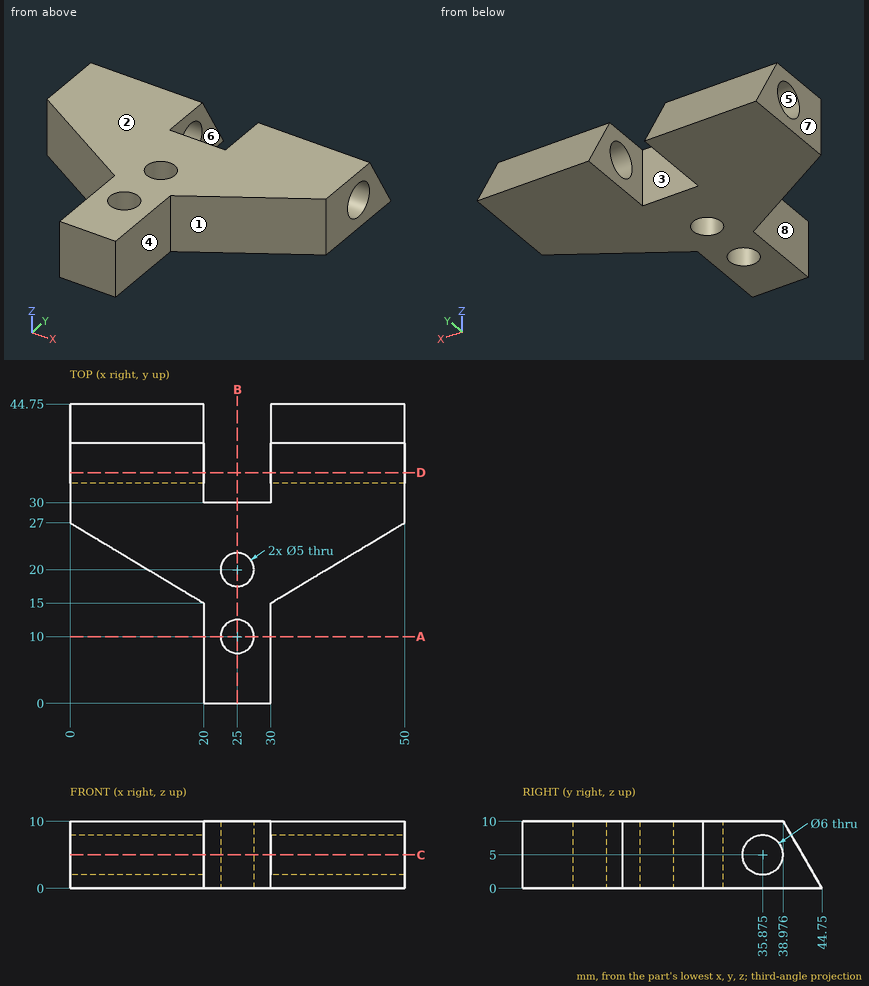
Study the drawing (mm; zero at the part's minimum x, y, z) and answer. A direction names the side the tool comes from. Round coordinates to 2 decimals unless told otherwise and drop trailing zeros. Write each loop counter-clockwise with the first axis right and the second up, starting at its lowest first coordinate (ties: lowest second). Pieces come first, ordered by that corner, then holes.
Q1. A tool of negligible diameter and unlimited length cuts with its end or side. For the marked faces 4, 5, 6, 7 and 8, from which of +Z, -Z, +X, -X, +Y, -Y can it reach the whole face along a straight path? Write none if from no direction.
Values:
face 4: +Z, -Z, +X, -Y
face 5: +X, -X
face 6: +Z, -Z, +Y
face 7: +Z, -Z, -X, +Y, -Y
face 8: +Z, -Z, -X, -Y
Q2. The mould has two halves that part along X. Classify the marked faces 1, 2 and 3: released by +X, released by -X, zero draft, split by the parting line, or undercut.
Values:
face 1: released by +X
face 2: zero draft
face 3: undercut
Q3. Find section C-C on z = 5. Determine the outline of the cut face in (x, y) (1 decimal).
Values:
outline: (0, 27) - (20, 15) - (20, 0) - (30, 0) - (30, 15) - (50, 27) - (50, 32.9) - (30, 32.9) - (30, 30) - (20, 30) - (20, 32.9) - (0, 32.9) - close; (0, 38.9) - (20, 38.9) - (20, 41.9) - (0, 41.9) - close; (30, 38.9) - (50, 38.9) - (50, 41.9) - (30, 41.9) - close; hole circle Ø5 at (25, 10); hole circle Ø5 at (25, 20)
Q4. Flat-ended cylindrical pins translate along their axes: P1, Ø3, axis at x = 23.5, z = 5, coming from the +Y side; P2, Ø2, axis at y = 15, z = 8.5, coming from the +X side (1 decimal); P3, Ø5, axis at y = 10.5, z = 2.5, coming from the +X side. Find the tip coordinate at first contact, or state that the pin passes through.
Values:
P1: stops at y = 30
P2: stops at x = 31.7
P3: stops at x = 30
Q5. Find section D-D on y = 34.5. Determine the outline of the cut face in (x, z), and give its area (3 significant figures).
Values:
outline: (0, 0) - (20, 0) - (20, 2.33) - (0, 2.33) - close; (0, 7.67) - (20, 7.67) - (20, 10) - (0, 10) - close; (30, 0) - (50, 0) - (50, 2.33) - (30, 2.33) - close; (30, 7.67) - (50, 7.67) - (50, 10) - (30, 10) - close
area: 187 mm2
Q6. Find section B-B on x = 25. Determine the outline of the cut face in (y, z), and give its area (3 significant figures).
Values:
outline: (0, 0) - (7.5, 0) - (7.5, 10) - (0, 10) - close; (12.5, 0) - (17.5, 0) - (17.5, 10) - (12.5, 10) - close; (22.5, 0) - (30, 0) - (30, 10) - (22.5, 10) - close
area: 200 mm2
Q7. Straight lines are drawn through the part: line 1 (Y direction, x = 25, z = 7.25); line 2 (Y direction, x = 27, z = 8); line 3 (X direction, y = 7, z = 7). For each, find the intervals that lie inside material, in ascending order.
Values:
line 1: y = 0 to 7.5, 12.5 to 17.5, 22.5 to 30
line 2: y = 0 to 8.5, 11.5 to 18.5, 21.5 to 30
line 3: x = 20 to 30
Q8. Find section A-A on y = 10. Determine the outline of the cut face in (x, z).
Values:
outline: (20, 0) - (22.5, 0) - (22.5, 10) - (20, 10) - close; (27.5, 0) - (30, 0) - (30, 10) - (27.5, 10) - close
